Source: CAD feature listing. Evaluate the final solid. Frame: model axes, mm. Face numbers are marked on the shaded views. A direction names the side the tool comes from. Give positions to 0.01 mm unless a question says otherwise; leave off trailing zeros. Order: outer loops, then holes, each group sorted by start corner. A loop starts at its lowest first (then second) coordinate and runs counter-clockwise, first axis right, second up. Notation, with made-up numbers: (33.25, -19) - (73.25, -19) arc R35 ccw to (73.25, 20) - close; hole circle Ø3 at (-25.75, 75.5). An arc over 180 degrees is marked (long way). Write each question's results on one line, items separated by ' | '. Start each with the question number.
Item 1: Line query: line 1 along X through (y, z) = (3.5, 10); line 2 along Z through (x, y) = (36, 6); line 3 along Z through (x, y) = (69, 12.5). Output: solid intervals per line, ascending.
Item 2: Contact query for flat-ended pins moving along their axis: pin 1 Ø8 at (x, z) = (81, 20.5) entering from -Y; pin 2 Ø4 at (y, z) = (44, 33) entering from -X; pin 3 Ø4.5 at (x, z) = (36, 10) entering from +Y. Output: stop coordinate, or through.
Item 3: Section D-D on z = 44.5. Output: boundary loops of the cut face in (x, y).
Item 4: Section B-B on y = 24. Output: boundary loops of the cut face in (x, z).
Item 5: Set-up query: the marked faces 1, 2, 3, 4 and 5. Return all of +Z, -Z, +X, -X, +Y, -Y with unobstructed straight access to the full face (end or side cutting, diameter ignored); none if empty.
Item 6: Mould query, pull axis X, two halves, no side actions, for the marked faces 6, 7 and 8. Classes: released by +X, released by -X, zero draft, split by the parting line, or undercut.
Item 7: Section A-A on x = 43. Output: boundary loops of the cut face in (y, z), and give its area (3 significant figures).
Item 8: Section C-C on z = 28. Output: boundary loops of the cut face in (x, y), and give its area (3 significant figures).
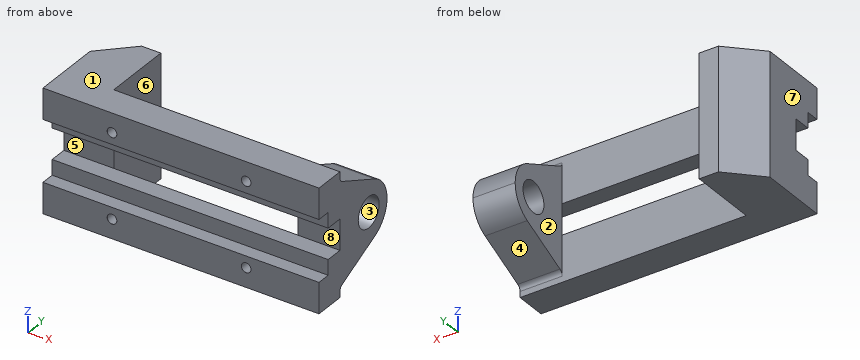
```python
from build123d import *

# Parameters (mm, degrees)
BOSS_EXTRUDE1_DEPTH                   = 64
CUT_EXTRUDE1_START                    = -22
CUT_EXTRUDE1_OUTLINE_R                = 8
CUT_EXTRUDE1_DEPTH                    = 22
CUT_EXTRUDE2_DEPTH                    = 166.939748102
TAP_DRILL_FOR_M6X1_0_TAP2_D           = 5
TAP_DRILL_FOR_M6X1_0_TAP2_DEPTH       = 10
TAP_DRILL_FOR_M6X1_0_TAP2_CSINK_D     = 5.05
TAP_DRILL_FOR_M6X1_0_TAP2_CSINK_ANGLE = 90
TAP_DRILL_FOR_M6X1_0_TAP2_TIP         = 1.502151548


# Read off the part's stored shape, not the designer's step: Cut-Extrude1
with BuildPart() as part:
    # Sketch1 → Boss-Extrude1 (new body)
    with BuildSketch(Plane.XY):
        Polygon((0, 0), (144, 0), (144, 16), (144, 52), (122, 52), (122, 16), (26, 16), (26, 52), (16, 52), (0, 36), (0, 16), align=None)
    extrude(amount=BOSS_EXTRUDE1_DEPTH)

    # Cut-Extrude1 outline → Cut-Extrude1 (cut)
    with BuildSketch(Plane(origin=(144, 0, 0), x_dir=(0, 0, -1), z_dir=(1, 0, 0)).offset(CUT_EXTRUDE1_START)):
        with BuildLine():
            ThreePointArc((-32, 52), (-23.403206266, 49.494263133), (-17.499075407, 42.761892188))
            Line((-17.499075407, 42.761892188), (-5.827512712, 17.732145215))
            ThreePointArc((-5.827512712, 17.732145215), (-4.720488176, 16.469825663), (-3.108589351, 16))
            Line((-3.108589351, 16), (0, 16))
            Line((0, 16), (0, 52))
            Line((0, 52), (-32, 52))
        make_face()
        with BuildLine():
            ThreePointArc((-46.500924593, 42.761892188), (-40.596793734, 49.494263133), (-32, 52))
            Line((-32, 52), (-64, 52))
            Line((-64, 52), (-64, 16))
            Line((-64, 16), (-60.891410649, 16))
            ThreePointArc((-60.891410649, 16), (-59.279511824, 16.469825663), (-58.172487288, 17.732145215))
            Line((-58.172487288, 17.732145215), (-46.500924593, 42.761892188))
        make_face()
        with Locations((-32, 38)):
            Circle(CUT_EXTRUDE1_OUTLINE_R)
    extrude(amount=CUT_EXTRUDE1_DEPTH, mode=Mode.SUBTRACT)

    # Sketch4_3 → Cut-Extrude2 (cut, through all)
    with BuildSketch(Plane(origin=(144, 0, 0), x_dir=(0, 0, -1), z_dir=(1, 0, 0))):
        Polygon((-24, 16), (-40, 16), (-40, 7), (-48, 7), (-48, 0), (-16, 0), (-16, 7), (-24, 7), align=None)
    extrude(amount=-CUT_EXTRUDE2_DEPTH, mode=Mode.SUBTRACT)

    # Tap Drill for M6x1.0 Tap2
    with Locations(Plane(origin=(0, 0, 0), x_dir=(-1, 0, 0), z_dir=(0, -1, 0))):
        with Locations((-36, -54), (-106, -54), (-106, -10), (-36, -10)):
            CounterSinkHole(TAP_DRILL_FOR_M6X1_0_TAP2_D / 2, TAP_DRILL_FOR_M6X1_0_TAP2_CSINK_D / 2, depth=TAP_DRILL_FOR_M6X1_0_TAP2_DEPTH, counter_sink_angle=TAP_DRILL_FOR_M6X1_0_TAP2_CSINK_ANGLE)
            with Locations((0, 0, -(TAP_DRILL_FOR_M6X1_0_TAP2_DEPTH + TAP_DRILL_FOR_M6X1_0_TAP2_TIP / 2))):  # 118° drill point
                Cone(0, TAP_DRILL_FOR_M6X1_0_TAP2_D / 2, TAP_DRILL_FOR_M6X1_0_TAP2_TIP, mode=Mode.SUBTRACT)


solid = part.part
```
Evaluation:
1) line 1: x = 0 to 33.5, 38.5 to 103.5, 108.5 to 144 | line 2: z = 0 to 7.5, 12.5 to 16, 48 to 51.5, 56.5 to 64 | line 3: z = 0 to 24, 40 to 64
2) pin 1: stops at y = 7 | pin 2: stops at x = 6 | pin 3: stops at y = 16
3) outline: (0, 7) - (144, 7) - (144, 45.99) - (122, 45.99) - (122, 16) - (26, 16) - (26, 52) - (16, 52) - (0, 36) - close
4) outline: (0, 0) - (26, 0) - (26, 64) - (0, 64) - close; (122, 8.75) - (144, 8.75) - (144, 55.25) - (122, 55.25) - close
5) face 1: +Z, +X, -X, +Y, -Y | face 2: +Z, -Z, +Y | face 3: +X | face 4: -Z, +X, +Y | face 5: +X, -X, -Y
6) face 6: undercut | face 7: released by -X | face 8: zero draft
7) outline: (0, 0) - (16, 0) - (16, 24) - (7, 24) - (7, 16) - (0, 16) - close; (0, 48) - (7, 48) - (7, 40) - (16, 40) - (16, 64) - (0, 64) - close | area: 656 mm^2
8) outline: (0, 16) - (26, 16) - (26, 52) - (16, 52) - (0, 36) - close; (122, 16) - (144, 16) - (144, 31.07) - (122, 31.07) - close; (122, 44.93) - (144, 44.93) - (144, 51.49) - (122, 51.49) - close | area: 1,280 mm^2
